CAD build for the part. Positions are in the model's coordinates, mm. Round coordinates to 2 decimals unless told otherwise and drop trailing zeros. Loops run counter-clockwise (first coordinate to the right, second up) from the corner with the lowest first, then second, coordinate; pieces in that order, holes last. Notation, with made-up numbers: M -1.5,27.25 L 38.5,27.25 A11 cw 38.5,47.25 Z; hole C 75.5,71 d2. An arc over 180 degrees is marked long. Use a Markdown table: item, result. Add a question column.
(1) Wall check: L1, parallel to X at y = 25, z = 7; L2, parallel to X at y = 22.5, z = 7; L3, parallel to Y at x = -85, z = 2.5. Give the ranges that are in metal, low to high.
(2) Band-saw the part on A-A, the plane x = -343. Write the cut outline in (y, z).
(3) Flat gauge pins, fed straight in: P1, Ø2, axis at y = 0.5, z = 4, coming from the -X side; P2, Ø3, axis at y = 4, z = 6, coming from the +X side; P3, Ø3, axis at x = 133, z = 2.5, coming from the +Y side; P4, Ø5, axis at x = 77, y = 34.5, coming from the +Z side. Where does each tip first touch, or does it go through?
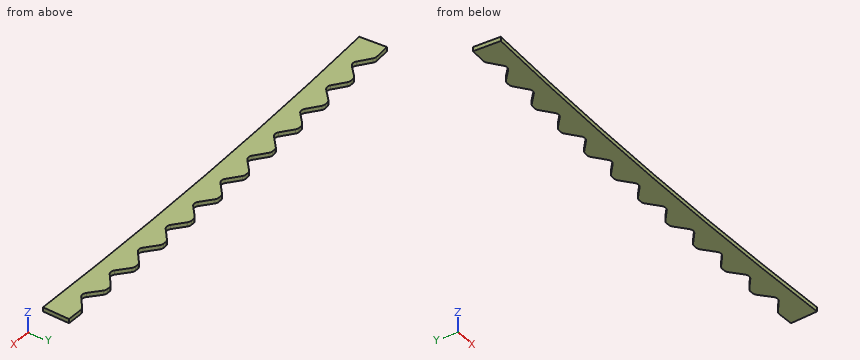
from build123d import *

# Parameters (mm, degrees)
BOSS_EXTRU_2_DEPTH                 = 8
ENL_V_MAT_EXTRU_1_DEPTH            = 9
CONG_1_R                           = 10
R_P_TITION_CIRCULAIRE1_COUNT       = 6
R_P_TITION_CIRCULAIRE1_ANGLE       = 2.3
CONG_1_OF_R_P_TITION_CIRCULAIRE1_R = 10
R_P_TITION_CIRCULAIRE2_COUNT       = 6
R_P_TITION_CIRCULAIRE2_ANGLE       = 2.3
CONG_1_OF_R_P_TITION_CIRCULAIRE2_R = 10


with BuildPart() as part:
    # Esquisse1 → Boss.-Extru.2 (new body)
    with BuildSketch(Plane.XY):
        with BuildLine():
            Line((423.958056387, -9.991125342), (426.313378922, 39.953368406))
            ThreePointArc((426.313378922, 39.953368406), (0, 50), (-426.313378922, 39.953368406))
            Line((-426.313378922, 39.953368406), (-423.958056387, -9.991125342))
            ThreePointArc((-423.958056387, -9.991125342), (0, 0), (423.958056387, -9.991125342))
        make_face()
    extrude(amount=BOSS_EXTRU_2_DEPTH)

    # Esquisse2 → Enlèv. mat.-Extru.1 (cut, through all)
    with BuildSketch(Plane.XY.offset(8)):
        Polygon((0, 25), (30, 49.950276106), (0, 74.995327729), (-30, 49.950276106), align=None)
    enl_v_mat_extru_1 = extrude(amount=-ENL_V_MAT_EXTRU_1_DEPTH, mode=Mode.SUBTRACT)

    # Congé1
    cong_1_edges = [part.edges().sort_by_distance(p)[0] for p in [
        (0, 25, 4),
        (-30, 49.950276106, 4),
        (30, 49.950276106, 4),
    ]]
    fillet(cong_1_edges, radius=CONG_1_R)

    # Répétition circulaire1: Enlèv. mat.-Extru.1 ×6 about axis
    r_p_tition_circulaire1_axis = Axis((0, -9000, 0), (0, 0, 1))
    for i in range(1, R_P_TITION_CIRCULAIRE1_COUNT):
        add(enl_v_mat_extru_1.rotate(r_p_tition_circulaire1_axis, i * R_P_TITION_CIRCULAIRE1_ANGLE / (R_P_TITION_CIRCULAIRE1_COUNT - 1)), mode=Mode.SUBTRACT)

    # Congé1 of Répétition circulaire1
    cong_1_of_r_p_tition_circulaire1_edges = [part.edges().sort_by_distance(p)[0] for p in [
        (-72.456565501, 24.709139142, 4),
        (-102.655910154, 49.417758293, 4),
        (-42.657843855, 49.899463992, 4),
        (-144.908460692, 23.836575317, 4),
        (-175.305203447, 48.301944876, 4),
        (-115.312938126, 49.265325224, 4),
        (-217.351015561, 22.382364766, 4),
        (-247.943197144, 46.602907776, 4),
        (-187.960599706, 48.047900678, 4),
        (-289.779560701, 20.346601223, 4),
        (-320.565209242, 44.320756509, 4),
        (-260.596145965, 46.247268824, 4),
        (-362.189427606, 17.729415908, 4),
        (-393.166558764, 41.455638174, 4),
        (-333.214895057, 43.863545726, 4),
    ]]
    fillet(cong_1_of_r_p_tition_circulaire1_edges, radius=CONG_1_OF_R_P_TITION_CIRCULAIRE1_R)

    # Répétition circulaire2: Enlèv. mat.-Extru.1 ×6 about axis
    r_p_tition_circulaire2_axis = Axis((0, -9000, 0), (0, 0, -1))
    for i in range(1, R_P_TITION_CIRCULAIRE2_COUNT):
        add(enl_v_mat_extru_1.rotate(r_p_tition_circulaire2_axis, i * R_P_TITION_CIRCULAIRE2_ANGLE / (R_P_TITION_CIRCULAIRE2_COUNT - 1)), mode=Mode.SUBTRACT)

    # Congé1 of Répétition circulaire2
    cong_1_of_r_p_tition_circulaire2_edges = [part.edges().sort_by_distance(p)[0] for p in [
        (72.456565501, 24.709139142, 4),
        (42.657843855, 49.899463992, 4),
        (102.655910154, 49.417758293, 4),
        (144.908460692, 23.836575317, 4),
        (115.312938126, 49.265325224, 4),
        (175.305203447, 48.301944876, 4),
        (217.351015561, 22.382364766, 4),
        (187.960599706, 48.047900678, 4),
        (247.943197144, 46.602907776, 4),
        (289.779560701, 20.346601223, 4),
        (260.596145965, 46.247268824, 4),
        (320.565209242, 44.320756509, 4),
        (362.189427606, 17.729415908, 4),
        (333.214895057, 43.863545726, 4),
        (393.166558764, 41.455638174, 4),
    ]]
    fillet(cong_1_of_r_p_tition_circulaire2_edges, radius=CONG_1_OF_R_P_TITION_CIRCULAIRE2_R)


solid = part.part
Return value:
| question | item | result |
|---|---|---|
| 1 | L1 | -425.61 to -371.68, -354.13 to -295.71, -284.69 to 284.69, 295.71 to 354.13, 371.68 to 425.61 |
| 1 | L2 | -425.49 to -368.4, -357.02 to 357.02, 368.4 to 425.49 |
| 1 | L3 | -0.4 to 34.97 |
| 2 | outline | M -6.54,0 L 35.04,0 L 35.04,8 L -6.54,8 Z |
| 3 | P1 | x = -424.5 |
| 3 | P2 | x = 424.69 |
| 3 | P3 | y = 35.36 |
| 3 | P4 | through |
